```python
from build123d import *

# Parameters (mm, degrees)
SKETCH_1_W          = 80
SKETCH_1_H          = 60
SKETCH_1_R          = 2.1
SKETCH_1_W_2        = 40
SKETCH_1_H_2        = 24
EXTRUDE_1_DEPTH     = 10
CUT_EXTRUDE_1_DEPTH = 80
CUT_EXTRUDE_2_DEPTH = 80
SKETCH_7_W          = 55
SKETCH_7_H          = 24
CUT_EXTRUDE_3_DEPTH = 1


with BuildPart() as part:
    # 草圖1 → 填料-伸長1 (new body)
    with BuildSketch(Plane(origin=(0, 0, 0), x_dir=(1, 0, 0), z_dir=(0, 1, 0))):
        Rectangle(SKETCH_1_W, SKETCH_1_H)
        with Locations(Location((-32.72, -5, 0), (0, 0, 270))):
            Circle(SKETCH_1_R, mode=Mode.SUBTRACT)
        with Locations(Location((-32.72, 5, 0), (0, 0, 270))):
            Circle(SKETCH_1_R, mode=Mode.SUBTRACT)
        with Locations(Location((13.48, -5, 0), (0, 0, 270))):
            Circle(SKETCH_1_R, mode=Mode.SUBTRACT)
        with Locations(Location((13.48, 5, 0), (0, 0, 270))):
            Circle(SKETCH_1_R, mode=Mode.SUBTRACT)
        with Locations((-9.62, 0)):
            Rectangle(SKETCH_1_W_2, SKETCH_1_H_2, mode=Mode.SUBTRACT)
    extrude(amount=EXTRUDE_1_DEPTH)

    # 草圖4 → 除料-伸長1 (cut)
    with BuildSketch(Plane(origin=(40, 0, 0), x_dir=(0, 0, -1), z_dir=(1, 0, 0))):
        Polygon((-23, 10), (-23, 8), (-25, 8), (-25, 3), (-15, 3), (-15, 8), (-17, 8), (-17, 10), align=None)
        Polygon((17, 10), (17, 8), (15, 8), (15, 3), (25, 3), (25, 8), (23, 8), (23, 10), align=None)
    extrude(amount=-CUT_EXTRUDE_1_DEPTH, mode=Mode.SUBTRACT)

    # 草圖5 → 除料-伸長2 (cut)
    with BuildSketch(Plane(origin=(0, 10, 0), x_dir=(1, 0, 0), z_dir=(0, 1, 0))):
        Polygon((10.38, 3.25), (13.63, 0), (10.38, -3.25), align=None)
    extrude(amount=-CUT_EXTRUDE_2_DEPTH, mode=Mode.SUBTRACT)

    # 草圖7 → 除料-伸長3 (cut)
    with BuildSketch(Plane(origin=(0, 10, 0), x_dir=(1, 0, 0), z_dir=(0, 1, 0))):
        with Locations((-9.62, 0)):
            Rectangle(SKETCH_7_W, SKETCH_7_H)
    extrude(amount=-CUT_EXTRUDE_3_DEPTH, mode=Mode.SUBTRACT)


solid = part.part
```
Build history of the part. All positions in model axes, mm. A direction names the side the tool comes from. Give positions to 0.01 mm unless a question says otherwise; leave off trailing zeros. Loops run counter-clockwise (first coordinate to the right, second up) from the corner with the lowest first, then second, coordinate; pieces in that order, holes last. Notation, with made-up numbers: (-3, 77.25) -> (16, 77.25) arc R30 ccw to (16, 111.25) -> close; hole circle Ø8 at (-33.5, 13.5). An arc over 180 degrees is marked (long way). One line per question, with ' | ' between items.
Q1. Drop flat-ended pins along their axis: pin 1 (2.5 mm diameter, centred on x = -32.72, z = 5, fed in from -Y); pin 2 (6 mm diameter, centred on x = 13.5, z = 5.5, fed in from +Y). Give the stop position or say it passes through.
Filled sheet:
pin 1: passes through | pin 2: stops at y = 9
Q2. Drill centre lines: line 1 along Z through (x, y) = (28, 5.75); line 2 along X through (y, z) = (4.75, 5); line 3 along Z through (x, y) = (6, 7.5). Where is each one in solid material? Low to high. Write a range as [from, to].
Filled sheet:
line 1: z = [-30, -25], [-15, 15], [25, 30] | line 2: x = [-40, -34.82], [-30.62, -29.62], [10.38, 11.38], [15.58, 40] | line 3: z = [-30, -25], [-15, -12], [12, 15], [25, 30]
Q3. Cut at C-C, the plane z = 5. Write the cut outline in (x, y).
Filled sheet:
outline: (-40, 0) -> (-34.82, 0) -> (-34.82, 9) -> (-37.12, 9) -> (-37.12, 10) -> (-40, 10) -> close; (-30.62, 0) -> (-29.62, 0) -> (-29.62, 9) -> (-30.62, 9) -> close; (10.38, 0) -> (11.38, 0) -> (11.38, 9) -> (10.38, 9) -> close; (15.58, 0) -> (40, 0) -> (40, 10) -> (17.88, 10) -> (17.88, 9) -> (15.58, 9) -> close
Q4. Cut at D-D, the plane x = -32.72. Count the separate pieces of the cut face and the enclosed holes in it, plus the area to 3 significant figures.
Filled sheet:
separate pieces: 3 | enclosed holes: 0 | area: 376 mm²
Q5. Cut at A-A, the plane y = 5. Write the cut outline in (x, z).
Filled sheet:
outline: (-40, -30) -> (40, -30) -> (40, -25) -> (-40, -25) -> close; (-40, -15) -> (40, -15) -> (40, 15) -> (-40, 15) -> close; (-40, 25) -> (40, 25) -> (40, 30) -> (-40, 30) -> close; hole circle Ø4.2 at (-32.72, -5); hole circle Ø4.2 at (-32.72, 5); hole (-29.62, -12) -> (10.38, -12) -> (10.38, -3.25) -> (13.63, 0) -> (10.38, 3.25) -> (10.38, 12) -> (-29.62, 12) -> close; hole circle Ø4.2 at (13.48, -5); hole circle Ø4.2 at (13.48, 5)
Q6. Pull direction X, two halves, no side cores. Call faces 1 (the flat face through (-1, 10, 26)), 2 (the flat face through (12.03, 4.56, 1.6)), 3 (the flat face through (40, 5, 0)): pulls with the +X half, pulls with the -X half, needs draft (parallel to the pull), parting line crosses it, or undercut.
Filled sheet:
face 1: needs draft | face 2: undercut | face 3: pulls with the +X half
Q7. Cut at B-B, the plane x = 3. Write the cut outline in (y, z).
Filled sheet:
outline: (0, -30) -> (10, -30) -> (10, -23) -> (8, -23) -> (8, -25) -> (3, -25) -> (3, -15) -> (8, -15) -> (8, -17) -> (10, -17) -> (10, -12) -> (0, -12) -> close; (0, 12) -> (10, 12) -> (10, 17) -> (8, 17) -> (8, 15) -> (3, 15) -> (3, 25) -> (8, 25) -> (8, 23) -> (10, 23) -> (10, 30) -> (0, 30) -> close
Q8. Tool access for faces 4 (the flat face through (1, 3, -20)), 5 (the flat face through (-29.62, 4, 0)), 6 (the flat face through (1, 9, 23)): list every direction of +Z, -Z, +X, -X, +Y, -Y with a clear straight run to the whole face (end or side of a thin tool).
Filled sheet:
face 4: +X, -X | face 5: +Y, -Y | face 6: +X, -X, +Y
